Work out the finished part from the listing and answer in its coordinate system (mm). Face numbers are marked on the shaded views. A direction names the side the tool comes from. Give positions to 0.01 mm unless a question says otherwise; leave off trailing zeros. Order: outer loops, then holes, each group sorted by start corner. A loop starts at its lowest first (then second) coordinate and runs counter-clockwise, first axis right, second up.
```python
from build123d import *

# Parameters (mm, degrees)
SKETCH1_W           = 55.372
SKETCH1_H           = 36.068
SKETCH1_R           = 3.175
BOSS_EXTRUDE1_DEPTH = 3.175
SKETCH2_W           = 3.175
SKETCH2_H           = 50.8
BOSS_EXTRUDE2_DEPTH = 38.1
CUT_EXTRUDE1_REACH  = 83.615
SKETCH3_R           = 3.175
CUT_EXTRUDE2_DEPTH  = 82.615263242


with BuildPart() as part:
    # Sketch1 → Boss-Extrude1 (new body)
    with BuildSketch(Plane(origin=(0, 0, 0), x_dir=(1, 0, 0), z_dir=(0, 1, 0))):
        with Locations((27.686, 18.034)):
            Rectangle(SKETCH1_W, SKETCH1_H)
        with Locations(Location((24.511, 8.89, 0), (0, 0, 270))):
            Circle(SKETCH1_R, mode=Mode.SUBTRACT)
        with Locations(Location((24.511, 26.162, 0), (0, 0, 270))):
            Circle(SKETCH1_R, mode=Mode.SUBTRACT)
        with Locations(Location((48.387, 8.89, 0), (0, 0, 270))):
            Circle(SKETCH1_R, mode=Mode.SUBTRACT)
    extrude(amount=BOSS_EXTRUDE1_DEPTH)

    # Sketch2 → Boss-Extrude2 (add)
    with BuildSketch(Plane(origin=(0, 3.175, 0), x_dir=(1, 0, 0), z_dir=(0, 1, 0))):
        with Locations((11.7475, 28.575)):
            Rectangle(SKETCH2_W, SKETCH2_H)
        with Locations((37.2745, 28.575)):
            Rectangle(SKETCH2_W, SKETCH2_H)
    extrude(amount=BOSS_EXTRUDE2_DEPTH)

    # Cut-Extrude1: up to this face of the body (flat: up to its plane)
    cut_extrude1_end = Plane(part.part.faces().sort_by_distance((38.862, 22.225, -28.575))[0])
    # Sketch3 → Cut-Extrude1 (cut, up to the picked face)
    with BuildSketch(Plane.ZY.offset(-10.16), mode=Mode.PRIVATE) as cut_extrude1_sk1:
        with Locations((-40.597508243, 23.435544859)):
            Circle(SKETCH3_R)
    cut_extrude1_tool1 = split(extrude(cut_extrude1_sk1.sketch, amount=-CUT_EXTRUDE1_REACH, mode=Mode.PRIVATE), bisect_by=cut_extrude1_end, keep=Keep.BOTH, mode=Mode.PRIVATE)
    add(cut_extrude1_tool1.solids().sort_by(Axis((10.16, 23.435545, -40.597508), (1, 0, 0)))[0], mode=Mode.SUBTRACT)

    # Sketch4 → Cut-Extrude2 (cut, through all)
    with BuildSketch(Plane.ZY.offset(-10.16)):
        with BuildLine():
            Line((-3.175, 3.175), (-3.175, 41.275))
            Line((-3.175, 41.275), (-53.975, 41.275))
            Line((-53.975, 41.275), (-53.975, 3.175))
            Line((-53.975, 3.175), (-36.068, 3.175))
            Line((-36.068, 3.175), (-49.342170052, 14.225719136))
            ThreePointArc((-49.342170052, 14.225719136), (-52.050540003, 28.923537523), (-38.898272892, 36.021354297))
            Line((-38.898272892, 36.021354297), (-9.300318539, 26.035))
            Line((-9.300318539, 26.035), (-3.175, 3.175))
        make_face()
    extrude(amount=-CUT_EXTRUDE2_DEPTH, mode=Mode.SUBTRACT)


solid = part.part
```
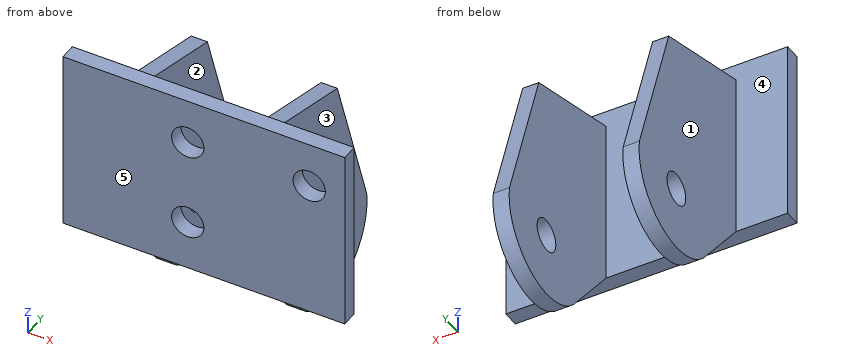
1. The part is cut by section B-B (x = 47). Write down the section's boundary in (y, z) (3 decimals), then the cut area to 3 significant figures.
Findings below:
outline: (0, -36.068) - (3.175, -36.068) - (3.175, -11.746) - (0, -11.746) - close; (0, -6.034) - (3.175, -6.034) - (3.175, 0) - (0, 0) - close
area: 96.4 mm2
2. The part is cut by section A-A (y = 17). Write down the section's boundary in (x, z) (3 decimals), then the cut area to 3 significant figures.
Findings below:
outline: (10.16, -51.546) - (13.335, -51.546) - (13.335, -6.879) - (10.16, -6.879) - close; (35.687, -51.546) - (38.862, -51.546) - (38.862, -6.879) - (35.687, -6.879) - close
area: 284 mm2
3. The mould has two halves that part along X. Classify the marked faces 3, 4 and 5: pulls with the +X half, pulls with the -X half, needs draft (parallel to the pull), parting line crosses it, or undercut.
Findings below:
face 3: pulls with the +X half
face 4: undercut
face 5: needs draft
4. Which of the six approach directions +Z, -Z, +X, -X, +Y, -Y give full straight-line access (tool end or side, diameter ignored) to the marked faces 1 and 2?
Findings below:
face 1: +Z, -Z, -X, +Y
face 2: +Z, -Z, +Y
5. The part is cut by section D-D (z = -16.5). Write down the section's boundary in (x, y) (3 decimals), then the cut area to 3 significant figures.
Findings below:
outline: (0, 0) - (55.372, 0) - (55.372, 3.175) - (38.862, 3.175) - (38.862, 28.464) - (35.687, 28.464) - (35.687, 3.175) - (13.335, 3.175) - (13.335, 28.464) - (10.16, 28.464) - (10.16, 3.175) - (0, 3.175) - close
area: 336 mm2
6. The part is cut by section C-C (y = 25). Write down the section's boundary in (x, z) (3 decimals).
Findings below:
outline: (10.16, -53.201) - (13.335, -53.201) - (13.335, -43.36) - (10.16, -43.36) - close; (10.16, -37.835) - (13.335, -37.835) - (13.335, -9.023) - (10.16, -9.023) - close; (35.687, -53.201) - (38.862, -53.201) - (38.862, -43.36) - (35.687, -43.36) - close; (35.687, -37.835) - (38.862, -37.835) - (38.862, -9.023) - (35.687, -9.023) - close
7. Given P1, Ø8.5, axis at x = 48.387, z = -8.89, coming from the -Y side; P2, Ø1, axis at x = 12.5, z = -40.5, coming from the -Y side; P3, Ø1.5, axis at y = 14, z = -7.5, coming from the +X side; P4, Ø1, axis at x = 28.5, y = 1.5, coming from the -Z side, each flat-ended and moving along its own axis, determine where each tip first touches the part or whether it passes through.
Findings below:
P1: stops at y = 0
P2: stops at y = 6.45
P3: stops at x = 38.86
P4: stops at z = -36.07
8. Straight lines are drawn through the part: probe 1 along X at (y, z) = (1.45, -8.89); probe 2 along X at (y, z) = (16.5, -16.5) (3 decimals); probe 3 along Y at (x, z) = (30, -18) (3 decimals). For each, find the intervals that lie inside material, in ascending order.
Findings below:
probe 1: x = 0 to 21.34, 27.69 to 45.21, 51.56 to 55.37
probe 2: x = 10.16 to 13.335, 35.687 to 38.862
probe 3: y = 0 to 3.175
